from build123d import *

# Parameters (mm, degrees)
F0_W          = 88.9
F0_H          = 88.9
F1_DEPTH      = 152.4
F1_DEPTH_BACK = 152.4
F2_R          = 38.9255
F3_DEPTH      = 16.51
F4_R          = 5.08


with BuildPart() as f1:
    # F0 (on Right) → F1 (new body, two sides)
    with BuildSketch(Plane.YZ) as f1_sk:
        Rectangle(F0_W, F0_H)
    extrude(amount=F1_DEPTH)
    extrude(f1_sk.sketch, amount=-F1_DEPTH_BACK)

    # F2 (on face) → F3 (cut)
    with BuildSketch(Plane.XY.offset(44.45)):
        with Locations((-107.95, 0)):
            Circle(F2_R)
        with Locations((25.4, 0)):
            Circle(F2_R)
    extrude(amount=-F3_DEPTH, mode=Mode.SUBTRACT)

    # F4
    f4_edges = [f1.edges().sort_by_distance(p)[0] for p in [
        (0, -44.45, 44.45),
        (0, 44.45, 44.45),
        (0, -44.45, -44.45),
        (0, 44.45, -44.45),
    ]]
    fillet(f4_edges, radius=F4_R)


solid = f1.part
Design review of the part built by this model. Coordinates are the model's own, in mm. A direction names the side the tool comes from. Round coordinates to 2 decimals unless told otherwise and drop trailing zeros. Write each loop counter-clockwise with the first axis right and the second up, starting at its lowest first coordinate (ties: lowest second). Pieces come first, ordered by that corner, then holes. Notation, with made-up numbers: (40, -26.75) - (86, -26.75) arc R33 ccw to (86, 7.25) - close; hole circle Ø6 at (52.5, 8.5). An arc over 180 degrees is marked (long way). Use a Markdown table: item, result. Add a question column.
1. Mouldability with a two-part tool opening along Y and no side actions: class faces 3 (the face through (-152.4, -1, 1)), 4 (the face through (2.134, -43.001, -42.922)), 5 (the face through (61.357, -14.909, 36.311)), 6 (the face through (2.134, 42.922, -43.001)) as +Y half, -Y half, draft (parallel to the pull), parting line (faces both ways), or undercut.
2. Wall thickness on probe 1 along Y at (x, z) = (25.4, 37.25); probe 2 along X at (y, z) = (-8.5, 35); probe 3 along Z at (x, y) = (6.5, 32): over which ranges is each line inside the solid? List them lowest first.
3. We need section B-B (y = 0). State the section outline as (x, z) points.
4. For faces 1 (the face through (2, 44.45, -1)), 2 (the face through (-71.993, -14.909, 36.311)), list the 3-axis set-ups (+Z, -Z, +X, -X, +Y, -Y) from which the entire face can be reached by the end or side of a thin tool; tool diameter is ignored.
5. We need section A-A (x = 25.4). State the section outline as (y, z) points, then the cut area to 3 significant figures.
Output:
| question | item | result |
|---|---|---|
| 1 | face 3 | draft |
| 1 | face 4 | -Y half |
| 1 | face 5 | undercut |
| 1 | face 6 | +Y half |
| 2 | probe 1 | y = -44.45 to -38.93, 38.93 to 44.45 |
| 2 | probe 2 | x = -152.4 to -145.94, -69.96 to -12.59, 63.39 to 152.4 |
| 2 | probe 3 | z = -44.45 to 27.94 |
| 3 | outline | (-152.4, -44.45) - (152.4, -44.45) - (152.4, 44.45) - (64.33, 44.45) - (64.33, 27.94) - (-13.53, 27.94) - (-13.53, 44.45) - (-69.02, 44.45) - (-69.02, 27.94) - (-146.88, 27.94) - (-146.88, 44.45) - (-152.4, 44.45) - close |
| 4 | face 1 | +Z, -Z, +X, -X, +Y |
| 4 | face 2 | +Z |
| 5 | outline | (-44.45, -39.37) arc R5.08 ccw to (-39.37, -44.45) - (39.37, -44.45) arc R5.08 ccw to (44.45, -39.37) - (44.45, 39.37) arc R5.08 ccw to (39.37, 44.45) - (38.93, 44.45) - (38.93, 27.94) - (-38.93, 27.94) - (-38.93, 44.45) - (-39.37, 44.45) arc R5.08 ccw to (-44.45, 39.37) - close |
| 5 | area | 6,600 mm2 |
